Check sheet for the drawn part. Datum: minimum x, y, z corner. Units: mm. Round coordinates to 2 decimals unless told otherwise and drop trailing zeros. Order: outer loops, then holes, each group sorted by start corner. A loop starts at its lowest first (then second) coordinate and runs counter-clockwise, first axis right, second up.
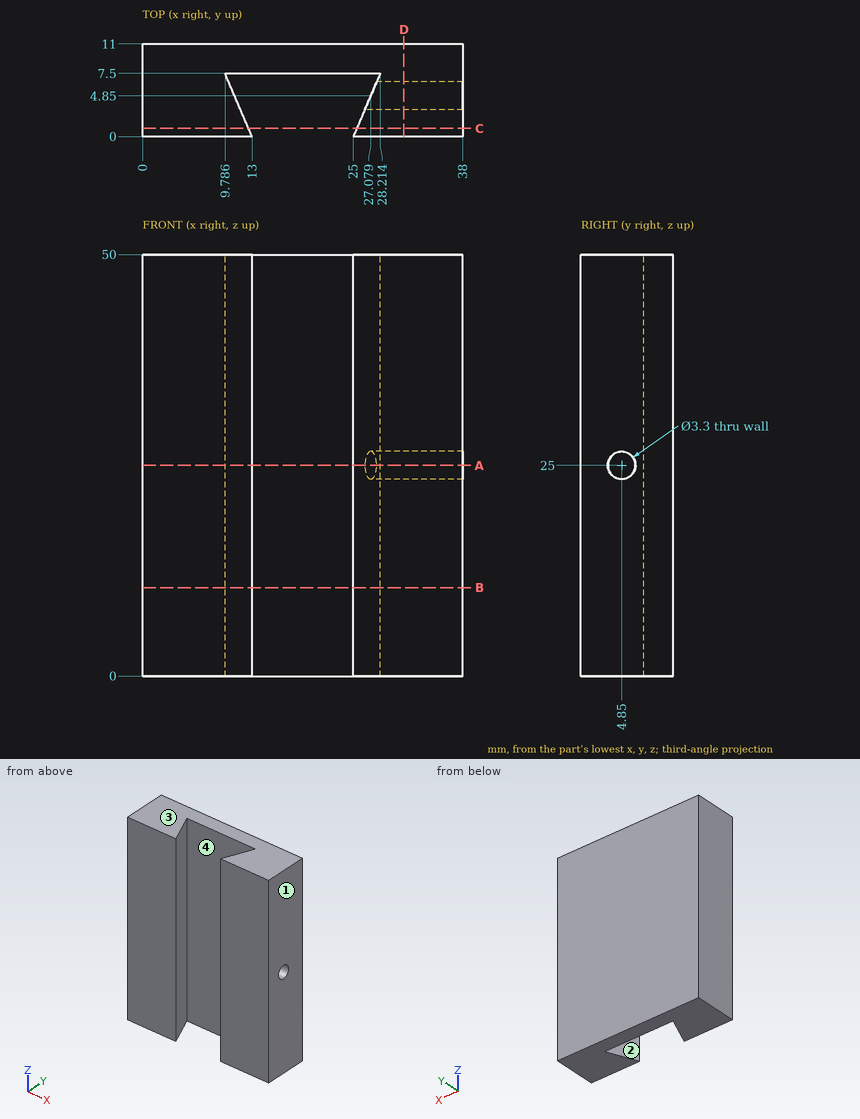
1) Draft check along X on the marked faces 1, 2, 3 and 4. Enter one of: pulls with the +X half, pulls with the -X half, needs draft (parallel to the pull), parting line crosses it, or undercut.
2) Scan lines: line 1 (Z direction, x = 30, y = 4.85); line 2 (Y direction, x = 29, z = 25); line 3 (X direction, y = 3, z = 46) (1 decimal). Record each from-to range of solid material in increasing order.
3) Sectioned sample at C-C on y = 1. Record the cut outline in (x, z), and give its area (3 significant figures).
4) Sectioned sample at B-B on z = 10.5. Record the cut outline in (x, y) (1 decimal).
5) Gauge pin test, flat end, axial feed: pin 1 (4 mm diameter, centred on x = 18.5, z = 24.5, fed in from -Y). Record the tip position at first contact, or that the pin passes through.
6) Sectioned sample at A-A on z = 25. Record the cut outline in (x, y) (1 decimal), and give its area (3 significant figures).
7) Sectioned sample at D-D on x = 31. Record the cut outline in (y, z).
Values found:
1. face 1: pulls with the +X half
1. face 2: undercut
1. face 3: needs draft
1. face 4: undercut
2. line 1: z = 0 to 23.35, 26.65 to 50
2. line 2: y = 0 to 3.2, 6.5 to 11
2. line 3: x = 0 to 11.7, 26.3 to 38
3. outline: (0, 0) - (12.57, 0) - (12.57, 50) - (0, 50) - close; (25.43, 0) - (38, 0) - (38, 50) - (25.43, 50) - close
3. area: 1,260 mm2
4. outline: (0, 0) - (13, 0) - (9.8, 7.5) - (28.2, 7.5) - (25, 0) - (38, 0) - (38, 11) - (0, 11) - close
5. pin 1: stops at y = 7.5
6. outline: (0, 0) - (13, 0) - (9.8, 7.5) - (28.2, 7.5) - (27.8, 6.5) - (38, 6.5) - (38, 11) - (0, 11) - close; (25, 0) - (38, 0) - (38, 3.2) - (26.4, 3.2) - close
6. area: 268 mm2
7. outline: (0, 0) - (11, 0) - (11, 50) - (0, 50) - close; hole circle Ø3.3 at (4.85, 25)
